Work out the finished part from the listing and answer in its coordinate system (mm). Face numbers are marked on the shaded views. A direction names the side the tool comes from. Coordinates: 2 decimals unless noted, no trailing zeros. Order: outer loops, then holes, each group sorted by start corner. A loop starts at its lowest first (then second) coordinate and runs counter-clockwise, first axis right, second up. Notation, with made-up numbers: (-17, -29.5) -> (29, -29.5) arc R35 cw to (29, 6.5) -> close; hole circle Ø9 at (62.25, 1). An arc over 180 degrees is marked (long way). Use one line per item in the form item = value.
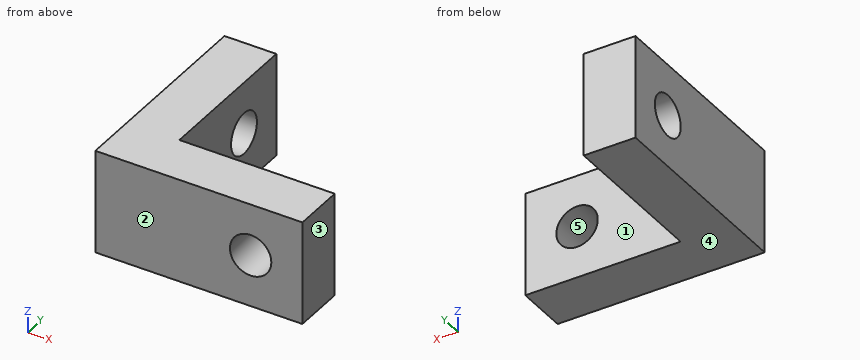
from build123d import *

# Parameters (mm, degrees)
SKETCH1_W           = 5
SKETCH1_H           = 15
SKETCH1_H_2         = 5
SKETCH1_W_2         = 15
BOSS_EXTRUDE2_DEPTH = 10
SKETCH3_R           = 2
CUT_EXTRUDE1_DEPTH  = 6
SKETCH4_R           = 2
CUT_EXTRUDE2_DEPTH  = 6


with BuildPart() as part:
    # Sketch1 → Boss-Extrude2 (new body)
    with BuildSketch(Plane.XY):
        with Locations((-7.340572317, 12.5)):
            Rectangle(SKETCH1_W, SKETCH1_H)
        with Locations((-7.340572317, 2.5)):
            Rectangle(SKETCH1_W, SKETCH1_H_2)
        with Locations((2.659427683, 2.5)):
            Rectangle(SKETCH1_W_2, SKETCH1_H_2)
    extrude(amount=BOSS_EXTRUDE2_DEPTH)

    # Sketch3 → Cut-Extrude1 (cut, through all)
    with BuildSketch(Plane(origin=(0, 5, 0), x_dir=(1, 0, 0), z_dir=(0, 1, 0))):
        with Locations((5.159427683, -5)):
            Circle(SKETCH3_R)
    extrude(amount=-CUT_EXTRUDE1_DEPTH, mode=Mode.SUBTRACT)

    # Sketch4 → Cut-Extrude2 (cut, through all)
    with BuildSketch(Plane(origin=(-4.840572317, 0, 0), x_dir=(0, 0, -1), z_dir=(1, 0, 0))):
        with Locations((-5, 15)):
            Circle(SKETCH4_R)
    extrude(amount=-CUT_EXTRUDE2_DEPTH, mode=Mode.SUBTRACT)


solid = part.part
(1) Section D-D on y = 3.5 is taken. Write down the section's boundary in (x, z), plus the area to 3 significant figures.
Data:
outline = (-9.84, 0) -> (10.16, 0) -> (10.16, 10) -> (-9.84, 10) -> close; hole circle Ø4 at (5.16, 5)
area = 187 mm²
(2) Section B-B on y = 15 is taken. Write down the section's boundary in (x, z), plus the area to 3 significant figures.
Data:
outline = (-9.84, 0) -> (-4.84, 0) -> (-4.84, 3) -> (-9.84, 3) -> close; (-9.84, 7) -> (-4.84, 7) -> (-4.84, 10) -> (-9.84, 10) -> close
area = 30.0 mm²
(3) Section A-A on z = 5 is taken. Write down the section's boundary in (x, y), plus the area to 3 significant figures.
Data:
outline = (-9.84, 0) -> (3.16, 0) -> (3.16, 5) -> (-4.84, 5) -> (-4.84, 13) -> (-9.84, 13) -> close; (-9.84, 17) -> (-4.84, 17) -> (-4.84, 20) -> (-9.84, 20) -> close; (7.16, 0) -> (10.16, 0) -> (10.16, 5) -> (7.16, 5) -> close
area = 135 mm²
(4) Straight lines are drawn through the part: line 1 along Y through (x, z) = (-6.4, 5); line 2 along X through (y, z) = (1.6, 5); line 3 along X through (y, z) = (8.75, 4.75). For each, find the intervals that lie inside material, in ascending order.
Data:
line_1 = 0 to 13, 17 to 20
line_2 = -9.84 to 3.16, 7.16 to 10.16
line_3 = -9.84 to -4.84
(5) The mould has two halves that part along X. Classify the marked faces 3, 4 and 5: released by +X, released by -X, zero draft, split by the parting line, or undercut.
Data:
face_3 = released by +X
face_4 = zero draft
face_5 = undercut
(6) Section C-C on x = -6.75 is taken. Write down the section's boundary in (y, z).
Data:
outline = (0, 0) -> (20, 0) -> (20, 10) -> (0, 10) -> close; hole circle Ø4 at (15, 5)
(7) Which of the six approach directions +Z, -Z, +X, -X, +Y, -Y give full straight-line access (tool end or side, diameter ignored) to the marked faces 1 and 2?
Data:
face_1 = +Z, -Z, +X, +Y
face_2 = +Z, -Z, +X, -X, -Y
(8) Each of these flat-tipped pins is pushed along its axis until it touches: P1, Ø3, axis at x = 1.5, z = 4.5, coming from the +Y side; P2, Ø3, axis at y = 13, z = 2.5, coming from the +X side; P3, Ø1.5, axis at x = -6.5, y = 11.5, coming from the -Z side. Where does it stop, or does it pass through?
Data:
P1 = 5
P2 = -4.84
P3 = 0
